```python
from build123d import *

# Parameters (mm, degrees)
F1_DEPTH = 3
F2_R     = 1


# Not quite as in the source:
# - a feature names something its author has since deleted; it is built from what else it names


with BuildPart() as f1:
    # F0 (on Top) → F1 (new body, symmetric)
    with BuildSketch(Plane.XY):
        with BuildLine():
            Line((-12.9470113486, 10.248668018), (-11.7864680784, 8.248668018))
            ThreePointArc((-11.7864680784, 8.248668018), (-7.2595115052, 2.3329471863), (-8.5698451786, -5))
            Line((-8.5698451786, -5), (-5.9368219527, -17.2248722292))
            ThreePointArc((-5.9368219527, -17.2248722292), (0, -16), (5.9368219527, -17.2248722292))
            Line((5.9368219527, -17.2248722292), (8.5698451786, -5))
            ThreePointArc((8.5698451786, -5), (7.2595115052, 2.3329471863), (11.7864680784, 8.248668018))
            Line((11.7864680784, 8.248668018), (12.9470113486, 10.248668018))
            Line((12.9470113486, 10.248668018), (10.9470113486, 10.248668018))
            ThreePointArc((10.9470113486, 10.248668018), (0, 7.2662124228), (-10.9470113486, 10.248668018))
            Line((-10.9470113486, 10.248668018), (-12.9470113486, 10.248668018))
        make_face()
    extrude(amount=F1_DEPTH, both=True)

    # F2
    f2_edges = [f1.edges().sort_by_distance(p)[0] for p in [
        (-12.947011, 10.248668, 0),
        (12.947011, 10.248668, 0),
        (-8.569845, -5, 0),
        (8.569845, -5, 0),
        (11.786468, 8.248668, 0),
        (-11.786468, 8.248668, 0),
    ]]
    fillet(f2_edges, radius=F2_R)


solid = f1.part
```
Design review of the part built by this model. Coordinates are the model's own, in mm. Give positions to 0.01 mm unless a question says otherwise; leave off trailing zeros. Order: outer loops, then holes, each group sorted by start corner. A loop starts at its lowest first (then second) coordinate and runs counter-clockwise, first axis right, second up. Notation, with made-up numbers: (20.5, -17.75) -> (72.5, -17.75) arc R19 cw to (72.5, 3.25) -> close; hole circle Ø10 at (63, 85). An arc over 180 degrees is marked (long way). Write item = value, one per line. Start each with the question number.
(1) For pin 1 (3 mm diameter, centred on x = 5.5, z = -2.5, fed in from -Y), flat-tipped, find the tip position at first contact; note if it passes through.
(2) We need section A-A on x = -7.5. Write out the cut boundary in (y, z), plus the area to 3 significant figures.
(3) To check wall thickness, follow line 1 along Y through (x, z) = (-0.25, 1.9); line 2 along X through (y, z) = (-6, 0.8); line 3 along X through (y, z) = (-11, -1.95). State the ranges of each line that lie inside material, in increasing order.
(4) We need section C-C on y = -10.5. Write out the cut boundary in (x, z), plus the area to 3 significant figures.
(5) We need section B-B on z = -2.4. Write out the cut boundary in (x, y), plus the area to 3 significant figures.
(6) We need section D-D on x = -0.25. Write out the cut boundary in (y, z), plus the area to 3 significant figures.
(7) Mouldability with a two-part tool opening along X and no side actions: class faces 1 (the face through (12.07, 9.76, 0.04)), 2 (the face through (-12.084, 9.735, -0.042)), 3 (the face through (0, -3, -3)), 4 (the face through (0.161, 7.267, 0.042)) as +X half, -X half, draft (parallel to the pull), parting line (faces both ways), or undercut.
Numbers:
q1.pin_1 = -17.22
q2.outline = (-9.97, -3) -> (-2.85, -3) -> (-2.85, 3) -> (-9.97, 3) -> close; (3.16, -3) -> (8.61, -3) -> (8.61, 3) -> (3.16, 3) -> close
q2.area = 75.5 mm^2
q3.line_1 = -16 to 7.27
q3.line_2 = -8.35 to 8.35
q3.line_3 = -7.28 to 7.28
q4.outline = (-7.39, -3) -> (7.39, -3) -> (7.39, 3) -> (-7.39, 3) -> close
q4.area = 88.6 mm^2
q5.outline = (-12.08, 8.75) -> (-11.92, 8.48) arc R1 ccw to (-11.56, 8.12) arc R9.24 cw to (-8.36, -4.67) arc R1 ccw to (-8.48, -5.4) -> (-5.94, -17.22) arc R15 cw to (5.94, -17.22) -> (8.48, -5.4) arc R1 ccw to (8.36, -4.67) arc R9.24 cw to (11.56, 8.12) arc R1 ccw to (11.92, 8.48) -> (12.08, 8.75) arc R1 ccw to (11.21, 10.25) -> (10.95, 10.25) arc R21.58 cw to (-10.95, 10.25) -> (-11.21, 10.25) arc R1 ccw to start
q5.area = 384 mm^2
q6.outline = (-16, -3) -> (7.27, -3) -> (7.27, 3) -> (-16, 3) -> close
q6.area = 140 mm^2
q7.face_1 = +X half
q7.face_2 = -X half
q7.face_3 = draft
q7.face_4 = undercut
